```python
from build123d import *

# Parameters (mm, degrees)
BOSS_EXTRU_4_DEPTH       = 25
BOSS_EXTRU_5_DEPTH       = 2.5
BOSS_EXTRU_6_DEPTH       = 5
ESQUISSE8_W              = 10
ESQUISSE8_H              = 10
ENL_V_MAT_EXTRU_3_DEPTH  = 10
ENL_V_START              = -25
ESQUISSE14_W             = 5
ESQUISSE14_H             = 3
ENL_V_MAT_EXTRU_13_DEPTH = 25
ENL_V_START_2            = -22
ESQUISSE15_W             = 3
ESQUISSE15_H             = 5
ENL_V_MAT_EXTRU_14_DEPTH = 22
BOSS_EXTRU_8_START       = -15
BOSS_EXTRU_8_DEPTH       = 15
BOSS_EXTRU_9_DEPTH       = 15
CONG_16_R                = 5
ESQUISSE20_R             = 2.5
ENL_V_MAT_EXTRU_16_DEPTH = 2
ENL_V_MAT_EXTRU_17_DEPTH = 3
CONG_31_R                = 1
CONG_37_R                = 1


with BuildPart() as part:
    # Esquisse1 → Boss.-Extru.4 (new body)
    with BuildSketch(Plane.XY):
        Polygon((-11.012370079, 11.844262295), (13.987629921, 11.844262295), (13.987629921, -13.155737705), (8.987629921, -13.155737705), (8.987629921, 6.844262295), (-11.012370079, 6.844262295), align=None)
    extrude(amount=BOSS_EXTRU_4_DEPTH)

    # Esquisse6 → Boss.-Extru.5 (add)
    with BuildSketch(Plane.XY.offset(25)):
        Polygon((10.987629921, -13.155737705), (13.987629921, -13.155737705), (13.987629921, 11.844262295), (-11.012370079, 11.844262295), (-11.012370079, 8.844262295), (10.987629921, 8.844262295), align=None)
    extrude(amount=BOSS_EXTRU_5_DEPTH)

    # Esquisse7 → Boss.-Extru.6 (add)
    with BuildSketch(Plane(origin=(0, 0, 0), x_dir=(-1, 0, 0), z_dir=(0, 0, -1))):
        Polygon((11.012370079, 6.844262295), (-8.987629921, -13.155737705), (-13.987629921, -13.155737705), (-13.987629921, 11.844262295), (11.012370079, 11.844262295), align=None)
    extrude(amount=BOSS_EXTRU_6_DEPTH)

    # Esquisse8 → Enlèv. mat.-Extru.3 (cut)
    with BuildSketch(Plane(origin=(13.987629921, 0, 0), x_dir=(0, 0, -1), z_dir=(1, 0, 0))):
        with Locations((-5, 6.844262295)):
            Rectangle(ESQUISSE8_W, ESQUISSE8_H)
    extrude(amount=-ENL_V_MAT_EXTRU_3_DEPTH, mode=Mode.SUBTRACT)

    # Esquisse14 → Enlèv. mat.-Extru.13 (cut)
    with BuildSketch(Plane.ZY.offset(11.012370079).offset(ENL_V_START)):
        with Locations((-2.5, 10.344262295)):
            Rectangle(ESQUISSE14_W, ESQUISSE14_H)
    extrude(amount=ENL_V_MAT_EXTRU_13_DEPTH, mode=Mode.SUBTRACT)

    # Esquisse15 → Enlèv. mat.-Extru.14 (cut)
    with BuildSketch(Plane(origin=(0, -13.155737705, 0), x_dir=(-1, 0, 0), z_dir=(0, -1, 0)).offset(ENL_V_START_2)):
        with Locations((-12.487629921, 2.5)):
            Rectangle(ESQUISSE15_W, ESQUISSE15_H)
    extrude(amount=ENL_V_MAT_EXTRU_14_DEPTH, mode=Mode.SUBTRACT)

    # Esquisse16 → Boss.-Extru.8 (add)
    with BuildSketch(Plane(origin=(0, -13.155737705, 0), x_dir=(-1, 0, 0), z_dir=(0, -1, 0)).offset(BOSS_EXTRU_8_START)):
        Polygon((-10.987629921, 0), (-13.987629921, 0), (-10.987629921, 5), align=None)
    extrude(amount=BOSS_EXTRU_8_DEPTH)

    # Esquisse17 → Boss.-Extru.9 (add)
    with BuildSketch(Plane.ZY.offset(11.012370079)):
        Polygon((-5, 8.844262295), (0, 11.844262295), (0, 8.844262295), align=None)
    extrude(amount=-BOSS_EXTRU_9_DEPTH)

    # Congé16
    cong_16_edges = [part.edges().sort_by_distance(p)[0] for p in [
        (13.987629921, 11.844262295, 18.75),
        (10.987629921, 8.844262295, -2.5),
    ]]
    fillet(cong_16_edges, radius=CONG_16_R)

    # Esquisse20 → Enlèv. mat.-Extru.16 (cut)
    with BuildSketch(Plane.XY.offset(-3)):
        with Locations((4.987629921, 2.844262295)):
            Circle(ESQUISSE20_R)
    extrude(amount=-ENL_V_MAT_EXTRU_16_DEPTH, mode=Mode.SUBTRACT)

    # Esquisse18 → Enlèv. mat.-Extru.17 (cut)
    with BuildSketch(Plane.XY):
        Polygon((2.129891888, -0.013475738), (6.033634639, -1.059480456), (8.891372672, 1.798257578), (7.845367954, 5.702000328), (3.941625204, 6.748005046), (1.08388717, 3.890267013), align=None)
    extrude(amount=-ENL_V_MAT_EXTRU_17_DEPTH, mode=Mode.SUBTRACT)

    # Congé31
    cong_31_edges = [part.edges().sort_by_distance(p)[0] for p in [
        (8.987629921, 1.844262295, 5),
        (3.987629921, 6.844262295, 5),
    ]]
    fillet(cong_31_edges, radius=CONG_31_R)

    # Congé37
    cong_37_edges = [part.edges().sort_by_distance(p)[0] for p in [
        (-3.512370079, 11.844262295, 0),
        (13.987629921, -5.655737705, 0),
    ]]
    fillet(cong_37_edges, radius=CONG_37_R)


solid = part.part
```
Could you check a few things on this model? Use its own coordinates, in mm. A direction names the side the tool comes from. Round coordinates to 2 decimals unless told otherwise and drop trailing zeros. Loops run counter-clockwise (first coordinate to the right, second up) from the corner with the lowest first, then second, coordinate; pieces in that order, holes last. Notation, with made-up numbers: (77.25, 27) -> (109.25, 27) arc R31 ccw to (109.25, 55) -> close; hole circle Ø8 at (-13.5, -38.5). An arc over 180 degrees is marked (long way). One line per question, with ' | ' between items.
(1) If we section it at B-B on x = 8.25: List the corners of the cut face in (y, z) for me, and give its area (3 significant figures).
Model answer:
outline: (-12.42, -5) -> (8.3, -5) -> (8.3, 0) -> (4.19, 0) -> (4.19, -3) -> (1.16, -3) -> (1.16, 0) -> (-12.42, 0) -> close; (6.84, 10) -> (11.84, 10) -> (11.84, 27.5) -> (8.84, 27.5) -> (8.84, 25) -> (6.84, 25) -> close | area: 177 mm^2
(2) Thinking about a two-plate mould opening in X: for faces 6 (the face through (7.442, 0.349, -1.479)), 7 (the face through (-11.012, 9, 11)), 8 (the face through (1.6, 1.97, -1.48)), 9 (the face through (2, 0, -5)), which applies, released by +X, released by -X, zero draft, split by the parting line, or undercut?
Model answer:
face 6: undercut | face 7: released by -X | face 8: undercut | face 9: zero draft
(3) If we section it at A-A on z = 9.5: List the corners of the cut face in (x, y) for me.
Model answer:
outline: (-11.01, 6.84) -> (2.99, 6.84) arc R1 ccw to (3.99, 7.84) -> (3.99, 11.84) -> (-11.01, 11.84) -> close; (8.99, -13.16) -> (13.99, -13.16) -> (13.99, 1.84) -> (9.99, 1.84) arc R1 ccw to (8.99, 0.84) -> close
(4) If I drill on probe 1 along Z at (x, y) = (9.5, 3.5); probe 2 along Z at (x, y) = (5, -6); probe 3 along Y at (x, z) = (-2, 5.5), over which ranges is the centre line in solid material (lowest first)?
Model answer:
probe 1: z = -5 to 0, 10 to 25 | probe 2: z = -5 to 0 | probe 3: y = 6.84 to 11.84
(5) For faces 1 (the face through (8.988, -6, 12)), 2 (the face through (9.5, 7.4, -2.5)), 3 (the face through (9.29, 1.56, 5.07)), 4 (the face through (3.7, 7.14, 5.07)), 5 (the face through (5.921, 6.218, -1.479)), which set-ups out of +Z, -Z, +X, -X, +Y, -Y let a thin tool reach every point of the face, with its end or its side?
Model answer:
face 1: +Z, -X, -Y | face 2: -Z, +X, +Y | face 3: -X, +Y | face 4: +X, -Y | face 5: +Z
(6) For pin 1 Ø6 at (x, z) = (0.5, 6.5) entering from -Y; pin 2 Ø4 at (y, z) = (4.5, 15) entering from -X; pin 3 Ø1.2 at (y, z) = (9, 5) entering from +X, each with a flat end and sliding along its axis, tell me the tip position at first contact or that it passes through.
Model answer:
pin 1: stops at y = 6.84 | pin 2: stops at x = 8.99 | pin 3: stops at x = 3.99
(7) If we section it at C-C on y = -8.5: List the corners of the cut face in (x, z) for me, and give its area (3 significant figures).
Model answer:
outline: (4.33, -5) -> (10.99, -5) -> (13.85, -0.24) arc R1 ccw to (13.99, 0.28) -> (13.99, 27.5) -> (10.99, 27.5) -> (10.99, 25) -> (8.99, 25) -> (8.99, 0) -> (4.33, 0) -> close | area: 173 mm^2
(8) If we section it at D-D on z = 13: List the corners of the cut face in (x, y) for me.
Model answer:
outline: (-11.01, 6.84) -> (8.99, 6.84) -> (8.99, -13.16) -> (13.99, -13.16) -> (13.99, 6.84) arc R5 ccw to (8.99, 11.84) -> (-11.01, 11.84) -> close
